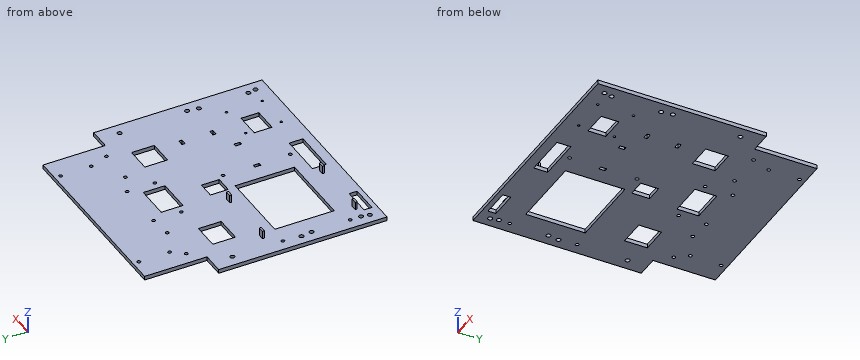
from build123d import *

# Parameters (mm, degrees)
EQUIPMENT_DECK_START                   = 32
EQUIPMENT_DECK_DEPTH                   = 4
EQUIPMENT_AND_CABLE_WINDOWS_START      = 31
SKETCH_EQUIPMENT_AND_CABLE_WINDOWS_W   = 28
SKETCH_EQUIPMENT_AND_CABLE_WINDOWS_H   = 8
SKETCH_EQUIPMENT_AND_CABLE_WINDOWS_W_2 = 44
SKETCH_EQUIPMENT_AND_CABLE_WINDOWS_H_2 = 14
SKETCH_EQUIPMENT_AND_CABLE_WINDOWS_W_3 = 25
SKETCH_EQUIPMENT_AND_CABLE_WINDOWS_H_3 = 18
SKETCH_EQUIPMENT_AND_CABLE_WINDOWS_W_4 = 75
SKETCH_EQUIPMENT_AND_CABLE_WINDOWS_H_4 = 60
SKETCH_EQUIPMENT_AND_CABLE_WINDOWS_W_5 = 17
SKETCH_EQUIPMENT_AND_CABLE_WINDOWS_H_5 = 23
SKETCH_EQUIPMENT_AND_CABLE_WINDOWS_W_6 = 27
SKETCH_EQUIPMENT_AND_CABLE_WINDOWS_W_7 = 34
SKETCH_EQUIPMENT_AND_CABLE_WINDOWS_H_6 = 22
EQUIPMENT_AND_CABLE_WINDOWS_DEPTH      = 6
CHASSIS_M4_START                       = 31
SKETCH_CHASSIS_M4_R                    = 2.25
CHASSIS_M4_DEPTH                       = 6
MID_POSTS_M4_START                     = 31
SKETCH_MID_POSTS_M4_R                  = 2.25
MID_POSTS_M4_DEPTH                     = 6
JETSON_CLAMPS_M3_START                 = 31
SKETCH_JETSON_CLAMPS_M3_R              = 1.7
JETSON_CLAMPS_M3_DEPTH                 = 6
MC02_M2_START                          = 31
SKETCH_MC02_M2_R                       = 1.15
MC02_M2_DEPTH                          = 6
XT_POSTS_M3_START                      = 31
SKETCH_XT_POSTS_M3_R                   = 1.7
XT_POSTS_M3_DEPTH                      = 6
DRIVER_TRAYS_M3_START                  = 31
SKETCH_DRIVER_TRAYS_M3_R               = 1.7
DRIVER_TRAYS_M3_DEPTH                  = 6
CAMERA_M3_START                        = 31
SKETCH_CAMERA_M3_R                     = 1.7
CAMERA_M3_DEPTH                        = 6
LOGIC_AND_FFC_STRAP_SLOTS_START        = 31
SKETCH_LOGIC_AND_FFC_STRAP_SLOTS_W     = 3.2
SKETCH_LOGIC_AND_FFC_STRAP_SLOTS_H     = 6
SKETCH_LOGIC_AND_FFC_STRAP_SLOTS_W_2   = 6
SKETCH_LOGIC_AND_FFC_STRAP_SLOTS_H_2   = 3.2
LOGIC_AND_FFC_STRAP_SLOTS_DEPTH        = 6
JETSON_LONGITUDINAL_STOPS_START        = 36
SKETCH_JETSON_LONGITUDINAL_STOPS_W     = 6
SKETCH_JETSON_LONGITUDINAL_STOPS_H     = 2
JETSON_LONGITUDINAL_STOPS_DEPTH        = 8


with BuildPart() as part:
    # Sketch_Equipment_deck → Equipment_deck (new body)
    with BuildSketch(Plane.XY.offset(EQUIPMENT_DECK_START)):
        Polygon((118, 85), (118, -85), (-118, -85), (-118, 85), (-96, 85), (-96, 148), (96, 148), (96, 85), align=None)
    extrude(amount=EQUIPMENT_DECK_DEPTH)

    # Sketch_Equipment_and_cable_windows → Equipment_and_cable_windows (cut)
    with BuildSketch(Plane.XY.offset(EQUIPMENT_AND_CABLE_WINDOWS_START)):
        with Locations((-85, -76)):
            Rectangle(SKETCH_EQUIPMENT_AND_CABLE_WINDOWS_W, SKETCH_EQUIPMENT_AND_CABLE_WINDOWS_H)
        with Locations((0, -68)):
            Rectangle(SKETCH_EQUIPMENT_AND_CABLE_WINDOWS_W_2, SKETCH_EQUIPMENT_AND_CABLE_WINDOWS_H_2)
        with Locations((63, -50)):
            Rectangle(SKETCH_EQUIPMENT_AND_CABLE_WINDOWS_W_3, SKETCH_EQUIPMENT_AND_CABLE_WINDOWS_H_3)
        with Locations((-50, -18)):
            Rectangle(SKETCH_EQUIPMENT_AND_CABLE_WINDOWS_W_4, SKETCH_EQUIPMENT_AND_CABLE_WINDOWS_H_4)
        with Locations((-6, 29)):
            Rectangle(SKETCH_EQUIPMENT_AND_CABLE_WINDOWS_W_5, SKETCH_EQUIPMENT_AND_CABLE_WINDOWS_H_3)
        with Locations((63, 58)):
            Rectangle(SKETCH_EQUIPMENT_AND_CABLE_WINDOWS_W_3, SKETCH_EQUIPMENT_AND_CABLE_WINDOWS_H_5)
        with Locations((-68, 60)):
            Rectangle(SKETCH_EQUIPMENT_AND_CABLE_WINDOWS_W_6, SKETCH_EQUIPMENT_AND_CABLE_WINDOWS_H_5)
        with Locations((0, 78)):
            Rectangle(SKETCH_EQUIPMENT_AND_CABLE_WINDOWS_W_7, SKETCH_EQUIPMENT_AND_CABLE_WINDOWS_H_6)
    extrude(amount=EQUIPMENT_AND_CABLE_WINDOWS_DEPTH, mode=Mode.SUBTRACT)

    # Sketch_Chassis_M4 → Chassis_M4 (cut)
    with BuildSketch(Plane.XY.offset(CHASSIS_M4_START)):
        with Locations(Location((-106.5, -65, 0), (0, 0, 180))):
            Circle(SKETCH_CHASSIS_M4_R)
        with Locations(Location((-106.5, -15, 0), (0, 0, 180))):
            Circle(SKETCH_CHASSIS_M4_R)
        with Locations(Location((-106.5, 65, 0), (0, 0, 180))):
            Circle(SKETCH_CHASSIS_M4_R)
        with Locations(Location((106.5, -65, 0), (0, 0, 180))):
            Circle(SKETCH_CHASSIS_M4_R)
        with Locations(Location((106.5, -15, 0), (0, 0, 180))):
            Circle(SKETCH_CHASSIS_M4_R)
        with Locations(Location((106.5, 65, 0), (0, 0, 180))):
            Circle(SKETCH_CHASSIS_M4_R)
    extrude(amount=CHASSIS_M4_DEPTH, mode=Mode.SUBTRACT)

    # Sketch_MID_posts_M4 → MID_posts_M4 (cut)
    with BuildSketch(Plane.XY.offset(MID_POSTS_M4_START)):
        with Locations(Location((-108, -73, 0), (0, 0, 180))):
            Circle(SKETCH_MID_POSTS_M4_R)
        with Locations(Location((-108, -4, 0), (0, 0, 180))):
            Circle(SKETCH_MID_POSTS_M4_R)
        with Locations(Location((108, -73, 0), (0, 0, 180))):
            Circle(SKETCH_MID_POSTS_M4_R)
        with Locations(Location((108, -4, 0), (0, 0, 180))):
            Circle(SKETCH_MID_POSTS_M4_R)
    extrude(amount=MID_POSTS_M4_DEPTH, mode=Mode.SUBTRACT)

    # Sketch_Jetson_clamps_M3 → Jetson_clamps_M3 (cut)
    with BuildSketch(Plane.XY.offset(JETSON_CLAMPS_M3_START)):
        with Locations(Location((-106.5, -54, 0), (0, 0, 180))):
            Circle(SKETCH_JETSON_CLAMPS_M3_R)
        with Locations(Location((-106.5, 14, 0), (0, 0, 180))):
            Circle(SKETCH_JETSON_CLAMPS_M3_R)
        with Locations(Location((6.5, -54, 0), (0, 0, 180))):
            Circle(SKETCH_JETSON_CLAMPS_M3_R)
        with Locations(Location((6.5, 14, 0), (0, 0, 180))):
            Circle(SKETCH_JETSON_CLAMPS_M3_R)
    extrude(amount=JETSON_CLAMPS_M3_DEPTH, mode=Mode.SUBTRACT)

    # Sketch_MC02_M2 → MC02_M2 (cut)
    with BuildSketch(Plane.XY.offset(MC02_M2_START)):
        with Locations(Location((53.8, -70, 0), (0, 0, 180))):
            Circle(SKETCH_MC02_M2_R)
        with Locations(Location((53.8, -34, 0), (0, 0, 180))):
            Circle(SKETCH_MC02_M2_R)
        with Locations(Location((89.8, -70, 0), (0, 0, 180))):
            Circle(SKETCH_MC02_M2_R)
        with Locations(Location((89.8, -34, 0), (0, 0, 180))):
            Circle(SKETCH_MC02_M2_R)
    extrude(amount=MC02_M2_DEPTH, mode=Mode.SUBTRACT)

    # Sketch_XT_posts_M3 → XT_posts_M3 (cut)
    with BuildSketch(Plane.XY.offset(XT_POSTS_M3_START)):
        with Locations(Location((-25, 73, 0), (0, 0, 180))):
            Circle(SKETCH_XT_POSTS_M3_R)
        with Locations(Location((-25, 101, 0), (0, 0, 180))):
            Circle(SKETCH_XT_POSTS_M3_R)
        with Locations(Location((25, 73, 0), (0, 0, 180))):
            Circle(SKETCH_XT_POSTS_M3_R)
        with Locations(Location((25, 101, 0), (0, 0, 180))):
            Circle(SKETCH_XT_POSTS_M3_R)
    extrude(amount=XT_POSTS_M3_DEPTH, mode=Mode.SUBTRACT)

    # Sketch_Driver_trays_M3 → Driver_trays_M3 (cut)
    with BuildSketch(Plane.XY.offset(DRIVER_TRAYS_M3_START)):
        with Locations(Location((-83, 99, 0), (0, 0, 180))):
            Circle(SKETCH_DRIVER_TRAYS_M3_R)
        with Locations(Location((-47, 99, 0), (0, 0, 180))):
            Circle(SKETCH_DRIVER_TRAYS_M3_R)
        with Locations(Location((45, 92, 0), (0, 0, 180))):
            Circle(SKETCH_DRIVER_TRAYS_M3_R)
        with Locations(Location((81, 92, 0), (0, 0, 180))):
            Circle(SKETCH_DRIVER_TRAYS_M3_R)
    extrude(amount=DRIVER_TRAYS_M3_DEPTH, mode=Mode.SUBTRACT)

    # Sketch_Camera_M3 → Camera_M3 (cut)
    with BuildSketch(Plane.XY.offset(CAMERA_M3_START)):
        with Locations(Location((-74, 111, 0), (0, 0, 180))):
            Circle(SKETCH_CAMERA_M3_R)
        with Locations(Location((-74, 142, 0), (0, 0, 180))):
            Circle(SKETCH_CAMERA_M3_R)
        with Locations(Location((74, 111, 0), (0, 0, 180))):
            Circle(SKETCH_CAMERA_M3_R)
        with Locations(Location((74, 142, 0), (0, 0, 180))):
            Circle(SKETCH_CAMERA_M3_R)
    extrude(amount=CAMERA_M3_DEPTH, mode=Mode.SUBTRACT)

    # Sketch_Logic_and_FFC_strap_slots → Logic_and_FFC_strap_slots (cut)
    with BuildSketch(Plane.XY.offset(LOGIC_AND_FFC_STRAP_SLOTS_START)):
        with Locations((5.8, -20)):
            Rectangle(SKETCH_LOGIC_AND_FFC_STRAP_SLOTS_W, SKETCH_LOGIC_AND_FFC_STRAP_SLOTS_H)
        with Locations((42.2, -20)):
            Rectangle(SKETCH_LOGIC_AND_FFC_STRAP_SLOTS_W, SKETCH_LOGIC_AND_FFC_STRAP_SLOTS_H)
        with Locations((68, -8.6)):
            Rectangle(SKETCH_LOGIC_AND_FFC_STRAP_SLOTS_W_2, SKETCH_LOGIC_AND_FFC_STRAP_SLOTS_H_2)
        with Locations((68, 22.6)):
            Rectangle(SKETCH_LOGIC_AND_FFC_STRAP_SLOTS_W_2, SKETCH_LOGIC_AND_FFC_STRAP_SLOTS_H_2)
    extrude(amount=LOGIC_AND_FFC_STRAP_SLOTS_DEPTH, mode=Mode.SUBTRACT)

    # Sketch_Jetson_longitudinal_stops → Jetson_longitudinal_stops (add)
    with BuildSketch(Plane.XY.offset(JETSON_LONGITUDINAL_STOPS_START)):
        with Locations((-92, -66.25)):
            Rectangle(SKETCH_JETSON_LONGITUDINAL_STOPS_W, SKETCH_JETSON_LONGITUDINAL_STOPS_H)
        with Locations((-30, -66.25)):
            Rectangle(SKETCH_JETSON_LONGITUDINAL_STOPS_W, SKETCH_JETSON_LONGITUDINAL_STOPS_H)
        with Locations((-92, 27.4)):
            Rectangle(SKETCH_JETSON_LONGITUDINAL_STOPS_W, SKETCH_JETSON_LONGITUDINAL_STOPS_H)
        with Locations((-30, 27.4)):
            Rectangle(SKETCH_JETSON_LONGITUDINAL_STOPS_W, SKETCH_JETSON_LONGITUDINAL_STOPS_H)
    extrude(amount=JETSON_LONGITUDINAL_STOPS_DEPTH)


solid = part.part
The model under review builds one solid part; all positions refer to its coordinate system, in mm. Coordinates: 2 decimals unless noted, no trailing zeros. Loops run counter-clockwise (first coordinate to the right, second up) from the corner with the lowest first, then second, coordinate; pieces in that order, holes last. Notation, with made-up numbers: (3.25, 63.5) -> (27.25, 63.5) arc R24 cw to (27.25, 94.5) -> close; hole circle Ø10 at (20.5, -1.5). An arc over 180 degrees is marked (long way). Use a Markdown table: item, result. Add a question column.
1. To check wall thickness, follow line 1 (Y direction, x = -80.5, z = 34); line 2 (Y direction, x = -47, z = 34.35); line 3 (Y direction, x = -25, z = 33.75). State the ranges of each line that lie inside material, in increasing order.
2. Clearance check with flat-ended pins moving along their axes: pin 1 Ø7 at (x, y) = (-108, -73) entering from +Z; pin 2 Ø6.5 at (x, z) = (-93, 41) entering from -Y; pin 3 Ø1 at (y, z) = (27, 41.5) entering from -X. State where each tip first meets the part, or that it passes through.
3. Add section B-B on x = 35. Write out the cut boundary in (y, z), plus the area to 3 significant figures.
4. Add section A-A on z = 38.5. Write out the cut boundary in (x, y), plus the area to 3 significant figures.
Returned:
| question | item | result |
|---|---|---|
| 1 | line 1 | y = -85 to -80, -72 to -48, 12 to 48.5, 71.5 to 148 |
| 1 | line 2 | y = -85 to -48, 12 to 97.3, 100.7 to 148 |
| 1 | line 3 | y = -85 to -48, 12 to 71.3, 74.7 to 99.3, 102.7 to 148 |
| 2 | pin 1 | stops at z = 36 |
| 2 | pin 2 | stops at y = -67.25 |
| 2 | pin 3 | stops at x = -95 |
| 3 | outline | (-85, 32) -> (148, 32) -> (148, 36) -> (-85, 36) -> close |
| 3 | area | 932 mm² |
| 4 | outline | (-95, -67.25) -> (-89, -67.25) -> (-89, -65.25) -> (-95, -65.25) -> close; (-95, 26.4) -> (-89, 26.4) -> (-89, 28.4) -> (-95, 28.4) -> close; (-33, -67.25) -> (-27, -67.25) -> (-27, -65.25) -> (-33, -65.25) -> close; (-33, 26.4) -> (-27, 26.4) -> (-27, 28.4) -> (-33, 28.4) -> close |
| 4 | area | 48.0 mm² |
